```python
from build123d import *

# Parameters (mm, degrees)
SKETCH1_R                      = 12.7
SKETCH1_R_2                    = 11.1125
EXTRUDE1_DEPTH                 = 152.4
CUT_EXTRUDE1_REACH             = 14.7
SKETCH2_W                      = 38.1
SKETCH2_H                      = 1.5875
CUT_EXTRUDE1_DIRECTION_2_REACH = 14.7


with BuildPart() as part:
    # Sketch1 → Extrude1 (new body)
    with BuildSketch(Plane.XY):
        Circle(SKETCH1_R)
        Circle(SKETCH1_R_2, mode=Mode.SUBTRACT)
    extrude(amount=EXTRUDE1_DEPTH)

    # Sketch2 → Cut-Extrude1 (cut, up to next)
    with BuildSketch(Plane(origin=(0, 0, 0), x_dir=(0, 0, -1), z_dir=(1, 0, 0)), mode=Mode.PRIVATE) as cut_extrude1_sk1:
        with Locations((-133.35, 0)):
            Rectangle(SKETCH2_W, SKETCH2_H)
    cut_extrude1_tool1 = extrude(cut_extrude1_sk1.sketch, amount=-CUT_EXTRUDE1_REACH, mode=Mode.PRIVATE) & part.part
    add(cut_extrude1_tool1.solids().sort_by_distance((0, 0, 133.35))[0], mode=Mode.SUBTRACT)

    # Sketch2 → Cut-Extrude1 direction 2 (cut, up to next)
    with BuildSketch(Plane(origin=(0, 0, 0), x_dir=(0, 0, -1), z_dir=(1, 0, 0)), mode=Mode.PRIVATE) as cut_extrude1_direction_2_sk1:
        with Locations((-133.35, 0)):
            Rectangle(SKETCH2_W, SKETCH2_H)
    cut_extrude1_direction_2_tool1 = extrude(cut_extrude1_direction_2_sk1.sketch, amount=CUT_EXTRUDE1_DIRECTION_2_REACH, mode=Mode.PRIVATE) & part.part
    add(cut_extrude1_direction_2_tool1.solids().sort_by_distance((0, 0, 133.35))[0], mode=Mode.SUBTRACT)


solid = part.part
```
Input: part model. Units: mm. Frame: model coordinates. Give positions to 0.01 mm unless a question says otherwise; leave off trailing zeros. Loops run counter-clockwise (first coordinate to the right, second up) from the corner with the lowest first, then second, coordinate; pieces in that order, holes last.
1) Section query C-C on z = 77.5. Return the cut outline in (x, y) (1 decimal).
A:
outline: circle Ø25.4 at (0, 0); hole circle Ø22.2 at (0, 0)
2) Contact query for flat-ended pins moving along their axis: pin 1 (4 mm diameter, centred on y = -3.5, z = 60.5, fed in from -X); pin 2 (0.8 mm diameter, centred on x = -12, z = 124, fed in from -Y); pin 3 (0.8 mm diameter, centred on x = -12, z = 125.5, fed in from +Y). Output: stop coordinate, or through.
A:
pin 1: stops at x = -12.61
pin 2: stops at y = -5.17
pin 3: stops at y = 5.17
3) Section query A-A on z = 138.5. Return the cut outline in (x, y) (1 decimal), and give its area (3 significant figures).
A:
outline: (-12.7, -0.8) arc R12.7 ccw to (12.7, -0.8) - (11.1, -0.8) arc R11.1 cw to (-11.1, -0.8) - close; (-12.7, 0.8) - (-11.1, 0.8) arc R11.1 cw to (11.1, 0.8) - (12.7, 0.8) arc R12.7 ccw to start
area: 114 mm2
4) Section query B-B on y = 4.25. Return the cut outline in (x, z), and give its area (3 significant figures).
A:
outline: (-11.97, 0) - (-10.27, 0) - (-10.27, 152.4) - (-11.97, 152.4) - close; (10.27, 0) - (11.97, 0) - (11.97, 152.4) - (10.27, 152.4) - close
area: 518 mm2
5) Line query: L1, parallel to X at y = 0, z = 31; L2, parallel to Y at x = -0.5, z = 29; L3, parallel to X at y = 10.25, z = 75. Output: solid intervals per line, ascending.
A:
L1: x = -12.7 to -11.11, 11.11 to 12.7
L2: y = -12.69 to -11.1, 11.1 to 12.69
L3: x = -7.5 to -4.29, 4.29 to 7.5
6) Mould query, pull axis X, two halves, no side actions, for faces 1 (the cylindrical face through (11.732, -4.864, 75.133)), 2 (the flat face through (0, -12, 152.4)), 3 (the cylindrical face through (10.265, -4.256, 75.133)). Classes: released by +X, released by -X, zero draft, split by the parting line, or undercut.
A:
face 1: split by the parting line
face 2: zero draft
face 3: undercut
